```python
from build123d import *

# Parameters (mm, degrees)
F0_W     = 101.6
F0_H     = 101.6
F1_DEPTH = 101.6
F2_R     = 25.4
F3_DEPTH = 101.6
F4_W     = 50.8
F4_H     = 50.8
F5_DEPTH = 50.8
F6_R     = 10.971648
F7_DEPTH = 101.6


with BuildPart() as f1:
    # F0 (on Front) → F1 (new body)
    with BuildSketch(Plane.XZ):
        with Locations((-50.8, 50.8)):
            Rectangle(F0_W, F0_H)
    extrude(amount=F1_DEPTH)

    # F2 (on face) → F3 (cut)
    with BuildSketch(Plane.XY.offset(101.6)):
        with Locations((-51.241014, -50.795451)):
            Circle(F2_R)
    extrude(amount=-F3_DEPTH, mode=Mode.SUBTRACT)

    # F4 (on face) → F5 (cut)
    with BuildSketch(Plane.YZ):
        with Locations((-76.2, 25.4)):
            Rectangle(F4_W, F4_H)
    extrude(amount=-F5_DEPTH, mode=Mode.SUBTRACT)

    # F6 (on face) → F7 (cut)
    with BuildSketch(Plane.XY.offset(101.6)):
        with Locations((-86.970754, -85.573204)):
            Circle(F6_R)
    extrude(amount=-F7_DEPTH, mode=Mode.SUBTRACT)


solid = f1.part
```
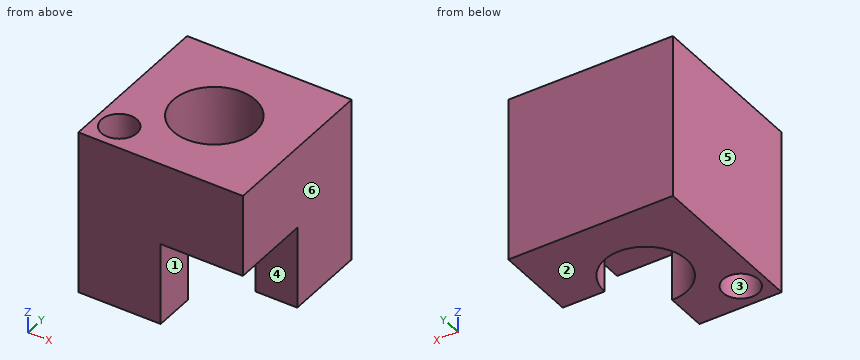
Check sheet for the modelled part. Datum: model origin and axes. Units: mm. Face numbers are marked on the shaded views. A direction names the side the tool comes from. Give positions to 0.01 mm unless a question says otherwise; leave off trailing zeros. Order: outer loops, then holes, each group sorted by start corner. A loop starts at its lowest first (then second) coordinate and runs counter-clockwise, first axis right, second up. Notation, with made-up numbers: M 34,72 L 60,72 A18 ccw 60,76 Z; hole C 56,40.25 d11. An arc over 180 degrees is marked long. Answer in a Markdown table with one row per item. Add a question column.
Q1. Thickness scan on L1, parallel to X at y = -85, z = 24; L2, parallel to Z at x = -26.5, y = -67; L3, parallel to X at y = -74, z = 86. Record the ranges inside material, lowest first.
Q2. Release check for a two-part mould opening along X. For the marked faces 3, 4, 5 and 6 record: released by +X, released by -X, zero draft, split by the parting line, or undercut.
Q3. Sectioned sample at D-D, the plane x = -17.5. Record the boundary of the cut face in (y, z), and give its area (3 significant figures).
Q4. Sectioned sample at A-A, the plane y = -81.5. Record the boundary of the cut face in (x, z).
Q5. Sectioned sample at B-B, the plane x = -68. Record the boundary of the cut face in (y, z).
Q6. Access from +Z, -Z, +X, -X, +Y, -Y to the whole of each face (thin tool, end or side, straight path). Record for the marked faces 1 and 2.
Q7. Gauge pin test, flat ends, axial feed: pin 1 Ø4 at (x, z) = (-37.5, 22) entering from -Y; pin 2 Ø13 at (x, z) = (-16.5, 20.5) entering from -Y; pin 3 Ø12.5 at (y, z) = (-93.5, 18.5) entering from +X; pin 4 Ø8 at (y, z) = (-53, 76.5) entering from +X. Record the tip position at first contact, or that the pin passes through.
Q8. Sectioned sample at C-C, the plane z = 43. Record the boundary of the cut face in (x, y), and give its area (3 significant figures).
Verdict:
| question | item | result |
|---|---|---|
| 1 | L1 | -101.6 to -97.93, -76.01 to -50.8 |
| 1 | L2 | 50.8 to 101.6 |
| 1 | L3 | -101.6 to -61.57, -40.91 to 0 |
| 2 | face 3 | undercut |
| 2 | face 4 | zero draft |
| 2 | face 5 | released by -X |
| 2 | face 6 | released by +X |
| 3 | outline | M -101.6,50.8 L -50.8,50.8 L -50.8,0 L 0,0 L 0,101.6 L -101.6,101.6 Z |
| 3 | area | 7,740 mm² |
| 4 | outline | M -101.6,0 L -97.16,0 L -97.16,101.6 L -101.6,101.6 Z; M -76.78,0 L -50.8,0 L -50.8,50.8 L 0,50.8 L 0,101.6 L -76.78,101.6 Z |
| 5 | outline | M -101.6,0 L -69.88,0 L -69.88,101.6 L -101.6,101.6 Z; M -31.71,0 L 0,0 L 0,101.6 L -31.71,101.6 Z |
| 6 | face 1 | -Z, +X, -Y |
| 6 | face 2 | -Z, +X, -X, +Y, -Y |
| 7 | pin 1 | y = -30.86 |
| 7 | pin 2 | y = -50.8 |
| 7 | pin 3 | x = -50.8 |
| 7 | pin 4 | x = 0 |
| 8 | outline | M -101.6,-101.6 L -50.8,-101.6 L -50.8,-76.19 A25.4 cw long -25.84,-50.8 L 0,-50.8 L 0,0 L -101.6,0 Z; hole C -86.97,-85.57 d21.94 |
| 8 | area | 5,830 mm² |
